Design review of the part built by this model. Coordinates are the model's own, in mm. Round coordinates to 2 decimals unless told otherwise and drop trailing zeros. Loops run counter-clockwise (first coordinate to the right, second up) from the corner with the lowest first, then second, coordinate; pieces in that order, holes last. Notation, with made-up numbers: (65.25, 60) -> (117.25, 60) arc R27 ccw to (117.25, 80) -> close; hole circle Ø11 at (9.5, 30). An arc over 180 degrees is marked (long way). Answer as CSV lines item,"result". Start each with the question number.
(1) Take a section at B-B, the plane y = 3.25. Write out the cut boundary in (x, z).
(2) Draft analysis for pull direction X (two halves, no side actions). For faces 1 (the face through (-1.5, 4.2, -0.07)), 2 (the face through (0.86, 7.26, 0.51)), 3 (the face through (0, 0, 0)), state which applies: +X half, -X half, draft (parallel to the pull), parting line (faces both ways), or undercut.
(3) Take a section at A-A, the plane x = 0. Write out the cut boundary in (y, z), and give its area (4 significant figures).
(4) To check wall thickness, follow line 1 (Y direction, x = 0.45, z = -0.25); line 2 (Z direction, x = 1.1, y = 7.5); line 3 (Z direction, x = 0.15, y = 5.25). State the ranges of each line that lie inside material, in increasing order. Write a range as from..to.
(5) For P1, Ø1.5, axis at x = -1, z = 0, coming from the -Y side, flat-tipped, find the tip position at first contact; note if it passes through.
from build123d import *

# Parameters (mm, degrees)
SKETCH1_R           = 1.5
BOSS_EXTRUDE1_DEPTH = 8
CHAMFER1_SIZE       = 0.5
CUT_EXTRUDE1_DEPTH  = 1.5


with BuildPart() as part:
    # Sketch1 → Boss-Extrude1 (new body)
    with BuildSketch(Plane(origin=(0, 0, 0), x_dir=(1, 0, 0), z_dir=(0, 1, 0))):
        Circle(SKETCH1_R)
    extrude(amount=BOSS_EXTRUDE1_DEPTH)

    # Chamfer1
    chamfer1_edges = [part.edges().sort_by_distance(p)[0] for p in [
        (-1.5, 0, 0),
    ]]
    chamfer(chamfer1_edges, length=CHAMFER1_SIZE)

    # Sketch2 → Cut-Extrude1 (cut)
    with BuildSketch(Plane(origin=(0, 8, 0), x_dir=(1, 0, 0), z_dir=(0, 1, 0))):
        Polygon((0.577350269, -1), (1.154700538, 0), (0.577350269, 1), (-0.577350269, 1), (-1.154700538, 0), (-0.577350269, -1), align=None)
    extrude(amount=-CUT_EXTRUDE1_DEPTH, mode=Mode.SUBTRACT)


solid = part.part
The answers:
1,outline,"circle Ø3 at (0, 0)"
2,face 1,"parting line"
2,face 2,"undercut"
2,face 3,"draft"
3,outline,"(0, -1) -> (0.5, -1.5) -> (8, -1.5) -> (8, -1) -> (6.5, -1) -> (6.5, 1) -> (8, 1) -> (8, 1.5) -> (0.5, 1.5) -> (0, 1) -> close"
3,area,"20.75 mm²"
4,line 1,"0..6.5"
4,line 2,"-1.02..-0.09, 0.09..1.02"
4,line 3,"-1.49..1.49"
5,P1,"y = 0"
